from build123d import *

# Parameters (mm, degrees)
SKETCH_1_W                 = 34
SKETCH_1_H                 = 40
EXTRUDE_273_DEPTH          = 13
SKETCH_2_R                 = 11
CUT_EXTRUDE_457_DEPTH      = 13
HOLE_WIZARD_M6_D           = 5.5
HOLE_WIZARD_M6_CSINK_D     = 10.4
HOLE_WIZARD_M6_CSINK_ANGLE = 90
FILLET_1404_R              = 5
CHAMFER_1_SIZE             = 1.5


with BuildPart() as part:
    # Эскиз1 → Extrude 273 (new body)
    with BuildSketch(Plane.XY):
        Rectangle(SKETCH_1_W, SKETCH_1_H)
    extrude(amount=-EXTRUDE_273_DEPTH)

    # Эскиз2 → Cut-Extrude 457 (cut)
    with BuildSketch(Plane.XY.offset(-13)):
        with Locations(Location((0, 0, 0), (0, 0, 180))):
            Circle(SKETCH_2_R)
    extrude(amount=CUT_EXTRUDE_457_DEPTH, mode=Mode.SUBTRACT)

    # КреплениеM6 (through all)
    with Locations(Plane.XY):
        with Locations((0, 15.5), (0, -15.5)):
            CounterSinkHole(HOLE_WIZARD_M6_D / 2, HOLE_WIZARD_M6_CSINK_D / 2, counter_sink_angle=HOLE_WIZARD_M6_CSINK_ANGLE)

    # Fillet 1404
    fillet_1404_edges = [part.edges().sort_by_distance(p)[0] for p in [
        (17, -20, -6.5),
        (-17, -20, -6.5),
        (-17, 20, -6.5),
        (17, 20, -6.5),
    ]]
    fillet(fillet_1404_edges, radius=FILLET_1404_R)

    # Фаска1
    # the kernel refuses this chamfer: 1.5 mm, written as the material it takes off along each edge
    with BuildSketch(Plane(origin=(-12, -15, 0), x_dir=(-1, 0, 0), z_dir=(0, 1, 0))) as chamfer_1_piece_1:
        Polygon((5 - CHAMFER_1_SIZE, 0), (5, -CHAMFER_1_SIZE), (5, 0), align=None)
    revolve(axis=Axis((-12, -15, 0), (0, 0, 1)), revolution_arc=90, mode=Mode.SUBTRACT)
    with BuildSketch(Plane(origin=(1.251761638, -20, 0), x_dir=(0, 0.9996219169112968, 0.02749587661058636), z_dir=(-1, 0, 0)), Plane(origin=(12, -20, 0), x_dir=(0, 0.9996219169112968, 0.02749587661058636), z_dir=(-1, 0, 0))) as chamfer_1_piece_2:
        Polygon((CHAMFER_1_SIZE * 0.999621916911, CHAMFER_1_SIZE * 0.0274958766106), (-CHAMFER_1_SIZE * 0.0274958766106, CHAMFER_1_SIZE * 0.999621916911), (0, 0), align=None)
    extrude(amount=13.251761638, mode=Mode.SUBTRACT)
    with BuildSketch(Plane(origin=(12, -15, 0), x_dir=(0, -1, 0), z_dir=(-1, 0, 0))) as chamfer_1_piece_3:
        Polygon((5 - CHAMFER_1_SIZE, 0), (5, -CHAMFER_1_SIZE), (5, 0), align=None)
    revolve(axis=Axis((12, -15, 0), (0, 0, 1)), revolution_arc=90, mode=Mode.SUBTRACT)
    with BuildSketch(Plane(origin=(17, 15, 0), x_dir=(-0.9996219169112968, 0, 0.02749587661058636), z_dir=(0, -1, 0)), Plane(origin=(-17, -15, 0), x_dir=(0.9996219169112968, 0, 0.02749587661058636), z_dir=(0, 1, 0))) as chamfer_1_piece_4:
        Polygon((CHAMFER_1_SIZE * 0.999621916911, CHAMFER_1_SIZE * 0.0274958766106), (-CHAMFER_1_SIZE * 0.0274958766106, CHAMFER_1_SIZE * 0.999621916911), (0, 0), align=None)
    extrude(amount=30, mode=Mode.SUBTRACT)
    with BuildSketch(Plane(origin=(12, 15, 0), x_dir=(0, 1, 0), z_dir=(-1, 0, 0))) as chamfer_1_piece_5:
        Polygon((5 - CHAMFER_1_SIZE, 0), (5, CHAMFER_1_SIZE), (5, 0), align=None)
    revolve(axis=Axis((12, 15, 0), (0, 0, -1)), revolution_arc=90, mode=Mode.SUBTRACT)
    with BuildSketch(Plane(origin=(-12, 20, 0), x_dir=(0, 0.027495876610586778, -0.9996219169112968), z_dir=(1, 0, 0)), Plane(origin=(-1.251761638, 20, 0), x_dir=(0, 0.027495876610586778, -0.9996219169112968), z_dir=(1, 0, 0))) as chamfer_1_piece_6:
        Polygon((CHAMFER_1_SIZE * 0.999621916911, -CHAMFER_1_SIZE * 0.0274958766106), (-CHAMFER_1_SIZE * 0.0274958766106, -CHAMFER_1_SIZE * 0.999621916911), (0, 0), align=None)
    extrude(amount=13.251761638, mode=Mode.SUBTRACT)
    with BuildSketch(Plane(origin=(-12, 15, 0), x_dir=(0, 1, 0), z_dir=(1, 0, 0))) as chamfer_1_piece_7:
        Polygon((5 - CHAMFER_1_SIZE, 0), (5, -CHAMFER_1_SIZE), (5, 0), align=None)
    revolve(axis=Axis((-12, 15, 0), (0, 0, 1)), revolution_arc=90, mode=Mode.SUBTRACT)


solid = part.part
Input: part model. Units: mm. Frame: model coordinates. Coordinates: 2 decimals unless noted, no trailing zeros. Loops run counter-clockwise (first coordinate to the right, second up) from the corner with the lowest first, then second, coordinate; pieces in that order, holes last.
(1) Material intervals for probe 1 along Y at (x, z) = (0, -6.5); probe 2 along Y at (x, z) = (-1, -1.75); probe 3 along Y at (x, z) = (-6, -9.5), sorted ascending.
(2) Section A-A on z = -8.25. Return the cut outline in (x, y), then the cut area to 3 significant figures.
(3) Section C-C on y = 0. Return the cut outline in (x, z), then the cut area to 3 significant figures.
(4) Section B-B on x = 0. Return the cut outline in (y, z).
(5) Section D-D on x = -8. Return the cut outline in (y, z), then the cut area to 3 significant figures.
(6) First-contact query: pin 1 Ø1 at (x, y) = (2.5, -10.5) entering from -Z; pin 2 Ø6.5 at (x, y) = (0, -15.5) entering from +Z; pin 3 Ø4.5 at (x, y) = (0, 15.5) entering from -Z. Flat tips, straight axial feed; report the tip coordinate or a pass-through.
Data:
1. probe 1: y = -20 to -18.25, -12.75 to -11, 11 to 12.75, 18.25 to 20
1. probe 2: y = -20 to -18.8, -12.2 to -10.95, 10.95 to 12.2, 18.8 to 20
1. probe 3: y = -20 to -9.22, 9.22 to 20
2. outline: (-17, -15) arc R5 ccw to (-12, -20) - (12, -20) arc R5 ccw to (17, -15) - (17, 15) arc R5 ccw to (12, 20) - (-12, 20) arc R5 ccw to (-17, 15) - close; hole circle Ø22 at (0, 0); hole circle Ø5.5 at (0, -15.5); hole circle Ø5.5 at (0, 15.5)
2. area: 911 mm2
3. outline: (-17, -13) - (-11, -13) - (-11, 0) - (-15.5, 0) - (-17, -1.5) - close; (11, -13) - (17, -13) - (17, -1.5) - (15.5, 0) - (11, 0) - close
3. area: 154 mm2
4. outline: (-20, -13) - (-18.25, -13) - (-18.25, -2.45) - (-19.6, -1.1) - (-20, -1.5) - close; (-12.75, -13) - (-11, -13) - (-11, -0.7) - (-12.75, -2.45) - close; (11, -13) - (12.75, -13) - (12.75, -2.45) - (11, -0.7) - close; (18.25, -13) - (20, -13) - (20, -1.5) - (19.6, -1.1) - (18.25, -2.45) - close
5. outline: (-20, -13) - (-7.55, -13) - (-7.55, 0) - (-18.5, 0) - (-20, -1.5) - close; (7.55, -13) - (20, -13) - (20, -1.5) - (18.5, 0) - (7.55, 0) - close
5. area: 321 mm2
6. pin 1: stops at z = -13
6. pin 2: stops at z = -1.95
6. pin 3: passes through
